Here's how the part is built. I have some questions about the finished solid (model axes, mm). A direction names the side the tool comes from. Give positions to 0.01 mm unless a question says otherwise; leave off trailing zeros. Loops run counter-clockwise (first coordinate to the right, second up) from the corner with the lowest first, then second, coordinate; pieces in that order, holes last.
Q1. Suppose I cut it at A-A (x = 46.5). List the corners of the cut face in (y, z) for me.
Q2. Suppose I cut it at C-C (y = -3). List the corners of the cut face in (x, z) for me.
Q3. Suppose I cut it at D-D (x = 38.5). List the corners of the cut face in (y, z) for me.
Q4. Thinking about a two-plate mould opening in Y: for faces 3 (the face through (10, -1.5, 0)), 4 (the face through (80, 0, 3)), 5 (the face through (39.44, -4.436, -2.307)), 6 (the face through (10, 1.5, 0)), which applies, pulls with the +Y half, pulls with the -Y half, needs draft (parallel to the pull), parting line crosses it, or undercut?
Q5. I'm going to push flat-ended pins straight in: P1, Ø1.5, axis at x = 63, y = -1.5, coming from the -Z side; P2, Ø3, axis at x = 14, y = 1.5, coming from the -Z side; P3, Ø6, axis at x = 21, y = 4, coming from the +Z side. Where does each tip first touch, or does it pass through?
Q6. I need wall thicknesses on probe 1 along Y at (x, z) = (8, -1.5); probe 2 along X at (y, z) = (-0.5, 3.5); probe 3 along Y at (x, z) = (27, -0.25). Which ranges of each line are inside material? Lowest first, please.
Q7. Suppose I cut it at B-B (z = -4). List the corners of the cut face in (x, y) for me.
Q8. For faces 1 (the face through (20, 0, 0)), 2 (the face through (80, 0, -3)), which set-ups out of +Z, -Z, +X, -X, +Y, -Y let a thin tool reach every point of the face, with its end or its side?
```python
from build123d import *

# Parameters (mm, degrees)
SKETCH_1_R          = 5
EXTRUDE_1_DEPTH     = 80
SKETCH_2_W          = 13.601077261
SKETCH_2_H          = 3
CUT_EXTRUDE_1_DEPTH = 20
CUT_EXTRUDE_2_DEPTH = 35


with BuildPart() as part:
    # 草图1 → 凸台-拉伸1 (new body)
    with BuildSketch(Plane(origin=(0, 0, 0), x_dir=(0, 0, -1), z_dir=(1, 0, 0))):
        Circle(SKETCH_1_R)
    extrude(amount=EXTRUDE_1_DEPTH)

    # 草图2 → 切除-拉伸1 (cut)
    with BuildSketch(Plane(origin=(0, 0, 0), x_dir=(0, 0, -1), z_dir=(1, 0, 0))):
        with Locations((0.220015061, 0)):
            Rectangle(SKETCH_2_W, SKETCH_2_H)
    extrude(amount=CUT_EXTRUDE_1_DEPTH, mode=Mode.SUBTRACT)

    # 草图3 → 切除-拉伸2 (cut)
    with BuildSketch(Plane(origin=(80, 0, 0), x_dir=(0, 0, -1), z_dir=(1, 0, 0))):
        Polygon((-0.999943638, -0.009058055), (-0.914206616, -12.008751766), (1.085793384, -11.994461897), (0.91431934, 12.004925525), (-1.08568066, 11.990635657), align=None)
    extrude(amount=-CUT_EXTRUDE_2_DEPTH, mode=Mode.SUBTRACT)


solid = part.part
```
Solutions:
1. outline: (-4.91, 0.96) - (4.89, 1.03) arc R5 ccw to start; (-4.89, -1.04) arc R5 ccw to (4.91, -0.97) - close
2. outline: (0, -4) - (80, -4) - (80, -1.02) - (45, -1.02) - (45, 0.98) - (80, 0.98) - (80, 4) - (0, 4) - close
3. outline: circle Ø10 at (0, 0)
4. face 3: undercut
4. face 4: needs draft
4. face 5: parting line crosses it
4. face 6: undercut
5. P1: stops at z = -4.94
5. P2: stops at z = -4.77
5. P3: stops at z = 4.9
6. probe 1: y = -4.77 to -1.5, 1.5 to 4.77
6. probe 2: x = 20 to 80
6. probe 3: y = -4.99 to 4.99
7. outline: (0, -3) - (80, -3) - (80, 3) - (0, 3) - (0, 1.5) - (20, 1.5) - (20, -1.5) - (0, -1.5) - close
8. face 1: +Z, -Z, -X
8. face 2: +Z, -Z, +X, +Y, -Y
